Print and shaded views of the part. All mm, measured from the part's lowest x, y and z. Round coordinates to 2 decimals unless told otherwise and drop trailing zeros. Write each loop counter-clockwise with the first axis right and the second up, starting at its lowest first coordinate (ties: lowest second). Pieces come first, ordered by that corner, then holes. Notation, with made-up numbers: (0, 52) -> (55, 52) arc R20 cw to (55, 65) -> close; hole circle Ø7 at (-36, 63.25). An arc over 180 degrees is marked (long way). Return JSON: item names as keys, results as strings. Group by question number.
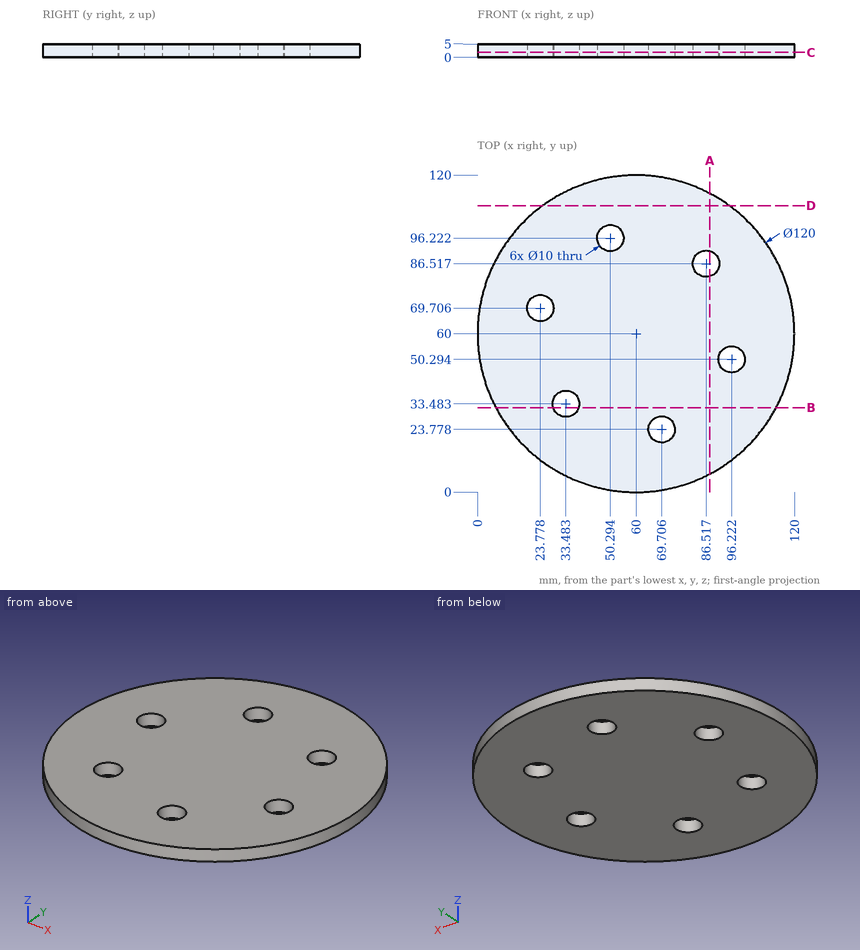
Item 1: Cut at D-D (y = 108.5). Write the cut outline in (x, z), then the cut area to 3 significant figures.
Item 2: Wall check: L1, parallel to Y at x = 68, z = 1.35 (1 decimal); L2, parallel to Y at x = 50, z = 3.9; L3, parallel to X at y = 38, z = 0.6 (1 decimal). Give the ranges that are in metal, low to high.
Item 3: Cut at C-C (z = 1.8). Write the cut outline in (x, y) (1 decimal), then the cut area to 3 significant figures.
Item 4: Cut at A-A (x = 88). Write the cut outline in (y, z) (1 decimal), then the cut area to 3 significant figures.
Item 5: Cut at B-B (y = 32). Write the cut outline in (x, z) (1 decimal), then the cut area to 3 significant figures.
Item 6: Flat gauge pins, fed straight in: P1, Ø6, axis at x = 55, y = 95.5, coming from the -Z side; P2, Ø1.5, axis at x = 80.5, z = 1, coming from the +Y side; P3, Ø1, axis at x = 83.5, z = 2.5, coming from the -Y side; P4, Ø8, axis at x = 96.22, y = 50.29, coming from the -Z side. Where does each tip first touch, or does it go through?
Checks:
{
 "1": {"outline": "(24.68, 0) -> (95.32, 0) -> (95.32, 5) -> (24.68, 5) -> close", "area": "353 mm2"},
 "2": {"L1": "y = 0.5 to 19.1, 28.5 to 119.5", "L2": "y = 0.84 to 91.23, 101.21 to 119.16", "L3": "x = 4.2 to 31.3, 35.6 to 115.8"},
 "3": {"outline": "circle Ø120 at (60, 60); hole circle Ø10 at (23.8, 69.7); hole circle Ø10 at (33.5, 33.5); hole circle Ø10 at (50.3, 96.2); hole circle Ø10 at (69.7, 23.8); hole circle Ø10 at (86.5, 86.5); hole circle Ø10 at (96.2, 50.3)", "area": "10,800 mm2"},
 "4": {"outline": "(6.9, 0) -> (81.7, 0) -> (81.7, 5) -> (6.9, 5) -> close; (91.3, 0) -> (113.1, 0) -> (113.1, 5) -> (91.3, 5) -> close", "area": "483 mm2"},
 "5": {"outline": "(6.9, 0) -> (28.7, 0) -> (28.7, 5) -> (6.9, 5) -> close; (38.3, 0) -> (113.1, 0) -> (113.1, 5) -> (38.3, 5) -> close", "area": "483 mm2"},
 "6": {"P1": "stops at z = 0", "P2": "stops at y = 116.66", "P3": "stops at y = 4.58", "P4": "passes through"}
}
